```python
from build123d import *

# Parameters (mm, degrees)
F0_W          = 25
F0_H          = 25
F3_R          = 1
F4_R          = 5
F5_DEPTH      = 12.5010001
F5_DEPTH_BACK = 12.5010001


with BuildPart() as f2:
    # F2: sweep along a path in F1
    with BuildLine(Plane.YZ) as f2_path:
        Line((0, 0), (0, -364.9896230895))
        ThreePointArc((0, -364.9896230895), (9.0423977856, -393.6684449071), (32.8989928337, -411.9742541288))
        Line((32.8989928337, -411.9742541288), (164.4462086375, -459.853525082))
    # F0 (on Top) → F2 (sweep)
    with BuildSketch(Plane.XY):
        Rectangle(F0_W, F0_H)
    sweep(path=f2_path.line)

    # F3
    f3_edges = [f2.edges().sort_by_distance(p)[0] for p in [
        (12.5, -12.5, -182.494812),
        (12.5, -1.197003, -400.83815),
        (-12.5, 94.397349, -447.660047),
        (12.5, 102.947853, -424.167732),
        (-12.5, 102.947853, -424.167732),
    ]]
    fillet(f3_edges, radius=F3_R)

    # F4 (on Right) → F5 (cut, two sides)
    with BuildSketch(Plane.YZ) as f5_sk:
        with Locations((0, -20)):
            Circle(F4_R)
        with Locations((0, -40)):
            Circle(F4_R)
        with Locations((0, -60)):
            Circle(F4_R)
        with Locations((0, -80)):
            Circle(F4_R)
        with Locations((0, -100)):
            Circle(F4_R)
        with Locations((0, -120)):
            Circle(F4_R)
        with Locations((0.1194545839, -140)):
            Circle(F4_R)
        with Locations((0, -160)):
            Circle(F4_R)
    extrude(amount=-F5_DEPTH, mode=Mode.SUBTRACT)
    extrude(f5_sk.sketch, amount=F5_DEPTH_BACK, mode=Mode.SUBTRACT)


solid = f2.part
```
For this review, take the finished solid that the model builds, in its own axes (mm). A direction names the side the tool comes from. Coordinates: 2 decimals unless noted, no trailing zeros. Loops run counter-clockwise (first coordinate to the right, second up) from the corner with the lowest first, then second, coordinate; pieces in that order, holes last.
1. Add section B-B, the plane z = -20. Give the boundary of the cut face in (x, y).
2. For line 1 (Y direction, x = 3.5, z = -60); line 2 (Y direction, x = -3.5, z = -308.5); line 3 (Z direction, x = 7, y = 17.5), list the stretches that pass through material, from the lowest coordinate up.
3. Add section A-A, the plane x = 5. Count the separate pieces of the cut face and the enclosed holes in it, then the cut area to 3 significant figures.
4. For faces 1 (the flat face through (0, 12.5, -185)), 2 (the cylindrical face through (12.215, 103.766, -424.785)), list the 3-axis set-ups (+Z, -Z, +X, -X, +Y, -Y) from which the entire face can be reached by the end or side of a thin tool; tool diameter is ignored.
5. Mouldability with a two-part tool opening along Y and no side actions: class faces 3 (the flat face through (12.5, 11, -271)), 4 (the cylindrical face through (0, 3, -116)), 5 (the flat face through (-0.161, 95.318, -447.995)), 6 (the cylindrical face through (0.175, 2.307, -164.436)) as +Y half, -Y half, draft (parallel to the pull), parting line (faces both ways), or undercut.
6. Insertion check: P1, Ø1, axis at x = 6, y = 128, coming from the -Z side; P2, Ø10, axis at x = 7.5, y = 45.5, coming from the +Z side; P3, Ø5, axis at x = -5.5, z = -373.5, coming from the +Y side. Each pin has a flat end and moves straight along its axis. Give the tip position at first contact, or say it passes through.
Result:
1. outline: (-12.5, -11.5) arc R1 ccw to (-11.5, -12.5) - (11.5, -12.5) arc R1 ccw to (12.5, -11.5) - (12.5, -5) - (-12.5, -5) - close; (-12.5, 5) - (12.5, 5) - (12.5, 11.5) arc R1 ccw to (11.5, 12.5) - (-11.5, 12.5) arc R1 ccw to (-12.5, 11.5) - close
2. line 1: y = -12.5 to -5, 5 to 12.5
2. line 2: y = -12.5 to 12.5
2. line 3: z = -418.38 to -383.7
3. separate pieces: 1
3. enclosed holes: 8
3. area: 13,500 mm2
4. face 1: +Z, +X, -X, +Y
4. face 2: +Z, +X, +Y
5. face 3: draft
5. face 4: undercut
5. face 5: -Y half
5. face 6: undercut
6. P1: stops at z = -460.07
6. P2: stops at z = -401.44
6. P3: stops at y = 14.15
